Work out the finished part from the listing and answer in its coordinate system (mm). A direction names the side the tool comes from. Give positions to 0.01 mm unless a question says otherwise; leave off trailing zeros. Loops run counter-clockwise (first coordinate to the right, second up) from the corner with the lowest first, then second, coordinate; pieces in that order, holes last.
from build123d import *

# Parameters (mm, degrees)
PAD025_DEPTH         = 120
POCKET029_DEPTH      = 2.101
SKETCH085_W          = 9.65
SKETCH085_H          = 4.8
PAD026_DEPTH         = 46
SKETCH086_R          = 1.75
POCKET030_DEPTH      = 46.001
SKETCH087_R          = 1.75
POCKET031_DEPTH      = 5.001
SKETCH088_R          = 3
POCKET032_DEPTH      = 2.951
POCKET043_DEPTH      = 49.401
SKETCH089_W          = 5.65
SKETCH089_H          = 2.75
POCKET033_DEPTH      = 35.151
POCKET033_DEPTH_BACK = 35.151
PAD027_DEPTH         = 2
PAD028_DEPTH         = 4


with BuildPart() as part:
    # Sketch083 → Pad025 (new body)
    with BuildSketch(Plane.YZ.offset(-21.698)):
        with BuildLine():
            ThreePointArc((-33.15, 1), (-32.857107, 0.292893), (-32.15, 0))
            Line((-32.15, 0), (32.15, 0))
            ThreePointArc((32.15, 0), (32.857107, 0.292893), (33.15, 1))
            Line((33.15, 1), (33.15, 46))
            Line((33.15, 46), (35.15, 46))
            Line((35.15, 46), (35.15, -2))
            Line((35.15, -2), (32.15, -5))
            Line((32.15, -5), (-32.15, -5))
            Line((-32.15, -5), (-35.15, -2))
            Line((-35.15, -2), (-35.15, 46))
            Line((-35.15, 46), (-33.15, 46))
            Line((-33.15, 46), (-33.15, 1))
        make_face()
    extrude(amount=PAD025_DEPTH)

    # Sketch084 → Pocket029 (cut, through all)
    with BuildSketch(Plane.YZ.offset(-19.598)):
        with BuildLine():
            ThreePointArc((-33.15, 1), (-32.857107, 0.292893), (-32.15, 0))
            Line((-32.15, 0), (32.15, 0))
            ThreePointArc((32.15, 0), (32.857107, 0.292893), (33.15, 1))
            Line((33.15, 46), (33.15, 1))
            Line((34.25, 46), (33.15, 46))
            Line((34.25, 1), (34.25, 46))
            ThreePointArc((32.15, -1.1), (33.634924, -0.484924), (34.25, 1))
            Line((-32.15, -1.1), (32.15, -1.1))
            ThreePointArc((-34.25, 1), (-33.634924, -0.484924), (-32.15, -1.1))
            Line((-34.25, 46), (-34.25, 1))
            Line((-33.15, 46), (-34.25, 46))
            Line((-33.15, 1), (-33.15, 46))
        make_face()
    extrude(amount=-POCKET029_DEPTH, mode=Mode.SUBTRACT)

    # Sketch085 → Pad026 (join)
    with BuildSketch(Plane.XY):
        with Locations((0, 30.75)):
            Rectangle(SKETCH085_W, SKETCH085_H)
        with Locations((60, 30.75)):
            Rectangle(SKETCH085_W, SKETCH085_H)
        with Locations((60, -30.75)):
            Rectangle(SKETCH085_W, SKETCH085_H)
        with Locations((0, -30.75)):
            Rectangle(SKETCH085_W, SKETCH085_H)
    extrude(amount=PAD026_DEPTH)

    # Sketch086 → Pocket030 (cut, through all)
    with BuildSketch(Plane.XY):
        with Locations((0, 31.75)):
            Circle(SKETCH086_R)
        with Locations((60, 31.75)):
            Circle(SKETCH086_R)
        with Locations((60, -31.75)):
            Circle(SKETCH086_R)
        with Locations((0, -31.75)):
            Circle(SKETCH086_R)
    extrude(amount=POCKET030_DEPTH, mode=Mode.SUBTRACT)

    # Sketch087 → Pocket031 (cut, through all)
    with BuildSketch(Plane.XY):
        with Locations((-15.348, 15.621)):
            Circle(SKETCH087_R)
        with Locations((-15.348, -19.431)):
            Circle(SKETCH087_R)
        with Locations((19.652, 0)):
            Circle(SKETCH087_R)
        with Locations((31.952, 15.621)):
            Circle(SKETCH087_R)
        with Locations((31.952, -19.431)):
            Circle(SKETCH087_R)
        with Locations((44.652, -19.431)):
            Circle(SKETCH087_R)
        with Locations((44.652, 15.621)):
            Circle(SKETCH087_R)
        with Locations((79.652, 0)):
            Circle(SKETCH087_R)
        with Locations((91.952, 15.621)):
            Circle(SKETCH087_R)
        with Locations((91.952, -19.431)):
            Circle(SKETCH087_R)
        with BuildLine():
            ThreePointArc((12.025, 28.35), (9.825, 30.550014), (7.625, 28.35))
            Line((7.625, 28.35), (7.625, 25.35))
            ThreePointArc((7.625, 25.35), (9.825, 18.009341), (12.025, 25.35))
            Line((12.025, 28.35), (12.025, 25.35))
        make_face()
        with BuildLine():
            ThreePointArc((12.025, -25.35), (9.825, -18.009341), (7.625, -25.35))
            Line((7.625, -25.35), (7.625, -28.35))
            ThreePointArc((7.625, -28.35), (9.825, -30.550011), (12.025, -28.35))
            Line((12.025, -25.35), (12.025, -28.35))
        make_face()
        with BuildLine():
            ThreePointArc((72.025, -25.35), (69.825, -18.009341), (67.625, -25.35))
            Line((67.625, -25.35), (67.625, -28.35))
            ThreePointArc((67.625, -28.35), (69.825, -30.550013), (72.025, -28.35))
            Line((72.025, -28.35), (72.025, -25.35))
        make_face()
        with BuildLine():
            ThreePointArc((72.025, 28.35), (69.825, 30.550019), (67.625, 28.35))
            Line((67.625, 25.35), (67.625, 28.35))
            ThreePointArc((67.625, 25.35), (69.825, 18.009341), (72.025, 25.35))
            Line((72.025, 28.35), (72.025, 25.35))
        make_face()
    extrude(amount=-POCKET031_DEPTH, mode=Mode.SUBTRACT)

    # Sketch088 → Pocket032 (cut, through all)
    with BuildSketch(Plane.XY.offset(-2.05)):
        with Locations((-15.348, 15.621)):
            Circle(SKETCH088_R)
        with Locations((-15.348, -19.431)):
            Circle(SKETCH088_R)
        with Locations((19.652, 0)):
            Circle(SKETCH088_R)
        with Locations((31.952, 15.621)):
            Circle(SKETCH088_R)
        with Locations((44.652, 15.621)):
            Circle(SKETCH088_R)
        with Locations((31.952, -19.431)):
            Circle(SKETCH088_R)
        with Locations((44.652, -19.431)):
            Circle(SKETCH088_R)
        with Locations((79.652, 0)):
            Circle(SKETCH088_R)
        with Locations((91.952, 15.621)):
            Circle(SKETCH088_R)
        with Locations((91.952, -19.431)):
            Circle(SKETCH088_R)
    extrude(amount=-POCKET032_DEPTH, mode=Mode.SUBTRACT)

    # Sketch111 → Pocket043 (cut, through all)
    with BuildSketch(Plane.XY.offset(-3.4)):
        with BuildLine():
            ThreePointArc((13.825, 28.35), (9.825, 32.350021), (5.825, 28.35))
            Line((5.825, 28.35), (5.825, 22.009341))
            Line((5.825, 22.009341), (13.825, 22.009341))
            Line((13.825, 22.009341), (13.825, 28.35))
        make_face()
        with BuildLine():
            ThreePointArc((73.825, 28.35), (69.825, 32.350007), (65.825, 28.35))
            Line((65.825, 28.35), (65.825, 22.009341))
            Line((65.825, 22.009341), (73.825, 22.009341))
            Line((73.825, 22.009341), (73.825, 28.35))
        make_face()
        with BuildLine():
            ThreePointArc((65.825, -28.349974), (69.824987, -32.350002), (73.825, -28.35))
            Line((73.825, -22.009341), (73.825, -28.35))
            Line((65.825, -22.009341), (73.825, -22.009341))
            Line((65.825, -28.349974), (65.825, -22.009341))
        make_face()
        with BuildLine():
            ThreePointArc((5.825, -28.349974), (9.824987, -32.350002), (13.825, -28.35))
            Line((13.825, -28.35), (13.825, -22.009341))
            Line((13.825, -22.009341), (5.825, -22.009341))
            Line((5.825, -22.009341), (5.825, -28.349974))
        make_face()
    extrude(amount=POCKET043_DEPTH, mode=Mode.SUBTRACT)

    # Sketch089 → Pocket033 (cut, two sides)
    with BuildSketch(Plane.XZ) as pocket033_sk:
        with Locations((0, 40.625)):
            Rectangle(SKETCH089_W, SKETCH089_H)
        with Locations((60, 40.625)):
            Rectangle(SKETCH089_W, SKETCH089_H)
    extrude(amount=-POCKET033_DEPTH, mode=Mode.SUBTRACT)
    extrude(pocket033_sk.sketch, amount=POCKET033_DEPTH_BACK, mode=Mode.SUBTRACT)

    # Sketch090 → Pad027 (join)
    with BuildSketch(Plane.YZ.offset(98.302)):
        with BuildLine():
            ThreePointArc((-33.15, 1), (-32.857107, 0.292893), (-32.15, 0))
            Line((-32.15, 0), (32.15, 0))
            ThreePointArc((32.15, 0), (32.857107, 0.292893), (33.15, 1))
            Line((33.15, 46), (33.15, 1))
            Line((34.05, 46), (33.15, 46))
            Line((34.05, 1), (34.05, 46))
            ThreePointArc((32.15, -0.9), (33.493503, -0.343503), (34.05, 1))
            Line((-32.15, -0.9), (32.15, -0.9))
            ThreePointArc((-34.05, 1), (-33.493503, -0.343503), (-32.15, -0.9))
            Line((-34.05, 46), (-34.05, 1))
            Line((-33.15, 46), (-34.05, 46))
            Line((-33.15, 1), (-33.15, 46))
        make_face()
    extrude(amount=PAD027_DEPTH)

    # Sketch091 → Pad028 (join)
    with BuildSketch(Plane.YZ.offset(100.302)):
        Polygon((-33.15, 46), (-28.35, 46), (-28.35, 36), (-33.15, 31.2), align=None)
        Polygon((33.15, 46), (28.35, 46), (28.35, 36), (33.15, 31.2), align=None)
    extrude(amount=-PAD028_DEPTH)


solid = part.part
Item 1: Find section B-B, the plane y = -10. Write down the section's boundary in (x, z), plus the area to 3 significant figures.
Item 2: Consider line 1 (X direction, y = -29.5, z = 35.5) (3 decimals); line 2 (X direction, y = 31.75, z = 44.45) (3 decimals); line 3 (Y direction, x = 51.5, z = 40.5). Determine where each line is inside the solid, lowest interval first.
Item 3: Find section C-C, the plane y = 0. Write down the section's boundary in (x, z).
Item 4: For faces 1 (the face through (0, 28.35, 23)), 2 (the face through (-4.825, -31, 23)), 3 (the face through (41.655, -19.299, -3.504)), 4 (the face through (61.669, 32.276, 19.35)), determine the directions among +Z, -Z, +X, -X, +Y, -Y from which every point of the face is accessible in a straight line to the end or side of a thin tool.
Item 5: Flat-ended cylindrical pins translate along their axes: pin 1 Ø1.8 at (y, z) = (26.5, -4.5) entering from +X; pin 2 Ø4 at (y, z) = (-31.5, 31.5) entering from -X; pin 3 Ø1.5 at (x, y) = (8.5, -17.5) entering from +Z. Find the tip coordinate at first contact, or state that the pin passes through.
Item 6: Find section A-A, the plane x = 0. Give the number of separate pieces and of enclosed holes in the cut face, plus the area to 3 significant figures.
Item 7: Determine the mould class of faces 5 (the face through (70, 31, -3.4)), 6 (the face through (62.825, -32, 41)), 7 (the face through (65.825, 25, -2)) for opening direction Z: released by +Z, released by -Z, zero draft, split by the parting line, or undercut.
Ans:
1. outline: (-21.7, -5) - (98.3, -5) - (98.3, -0.9) - (100.3, -0.9) - (100.3, 0) - (-19.6, 0) - (-19.6, -1.1) - (-21.7, -1.1) - close
1. area: 599 mm2
2. line 1: x = -4.825 to 4.825, 55.175 to 64.825, 96.302 to 100.302
2. line 2: x = -4.825 to -1.75, 1.75 to 4.825, 55.175 to 58.25, 61.75 to 64.825, 96.302 to 100.302
2. line 3: y = -35.15 to -33.15, 33.15 to 35.15
3. outline: (-21.7, -5) - (16.65, -5) - (16.65, -2.05) - (17.9, -2.05) - (17.9, 0) - (-19.6, 0) - (-19.6, -1.1) - (-21.7, -1.1) - close; (21.4, -2.05) - (22.65, -2.05) - (22.65, -5) - (76.65, -5) - (76.65, -2.05) - (77.9, -2.05) - (77.9, 0) - (21.4, 0) - close; (81.4, -2.05) - (82.65, -2.05) - (82.65, -5) - (98.3, -5) - (98.3, -0.9) - (100.3, -0.9) - (100.3, 0) - (81.4, 0) - close
4. face 1: +Z, +X, -X
4. face 2: +Z, -X
4. face 3: -Z
4. face 4: +Z
5. pin 1: stops at x = 98.3
5. pin 2: stops at x = -19.6
5. pin 3: stops at z = 0
6. separate pieces: 5
6. enclosed holes: 0
6. area: 628 mm2
7. face 5: released by +Z
7. face 6: undercut
7. face 7: zero draft
